```python
from build123d import *

# Parameters (mm, degrees)
SKETCH_1_R       = 2.9
EXTRUDE_1_DEPTH  = 4
CHAMFER_1_SIZE   = 0.6
SKETCH_3_W       = 12
SKETCH_3_H       = 19.86
EXTRUDE_2_DEPTH  = 2
SKETCH_4_W       = 10
SKETCH_4_H       = 12
SKETCH_4_R       = 1.6
EXTRUDE_3_DEPTH  = 3
FILLET_START     = -15
FILLET_2_DEPTH   = 4.14
FILLET_START_2   = -13.86
FILLET_2_2_DEPTH = 3
CHAMFER_4_SIZE   = 1


with BuildPart() as part:
    # 草图1 → 凸台-拉伸1 (new body)
    with BuildSketch(Plane.XY):
        Polygon((7.937253933, 6), (-21, 6), (-21, -13.86), (7.937253933, -13.86), (21, -13.86), (21, 6), align=None)
        Circle(SKETCH_1_R, mode=Mode.SUBTRACT)
    extrude(amount=EXTRUDE_1_DEPTH)

    # 倒角1
    chamfer_1_edges = [part.edges().sort_by_distance(p)[0] for p in [
        (-2.9, 0, 4),
    ]]
    chamfer(chamfer_1_edges, length=CHAMFER_1_SIZE)

    # 草图3 → 凸台-拉伸2 (add)
    with BuildSketch(Plane.ZY.offset(21)):
        with Locations((6, -3.93)):
            Rectangle(SKETCH_3_W, SKETCH_3_H)
    extrude_2 = extrude(amount=EXTRUDE_2_DEPTH)

    # 镜向1: 凸台-拉伸2 across plane
    add(extrude_2.mirror(Plane(origin=(0, 0, 0), x_dir=(0, 0, 1), z_dir=(1, 0, 0))))

    # 草图4 → 凸台-拉伸3 (add)
    # profile 1 of 2: a face of its own
    with BuildSketch(Plane.XZ.offset(13.86)):
        with Locations((-18, 6)):
            Rectangle(SKETCH_4_W, SKETCH_4_H)
        with Locations((-17, 8)):
            Circle(SKETCH_4_R, mode=Mode.SUBTRACT)
    # profile 2 of 2: a face of its own
    with BuildSketch(Plane.XZ.offset(13.86)):
        with Locations((18, 6)):
            Rectangle(SKETCH_4_W, SKETCH_4_H)
        with Locations(Location((17, 8, 0), (0, 0, 180))):
            Circle(SKETCH_4_R, mode=Mode.SUBTRACT)
    extrude(amount=-EXTRUDE_3_DEPTH)

    # 圆角2: read off the stored shape, not the designer's step
    # 圆角2 outline → 圆角2 (cut)
    with BuildSketch(Plane(origin=(0, 0, 0), x_dir=(1, 0, 0), z_dir=(0, 1, 0)).offset(FILLET_START)):
        with BuildLine():
            Line((13, -12), (17, -12))
            ThreePointArc((17, -12), (14.171572875, -10.828427125), (13, -8))
            Line((13, -8), (13, -12))
        make_face()
        with BuildLine():
            Line((-13, -12), (-13, -8))
            ThreePointArc((-13, -8), (-14.171572875, -10.828427125), (-17, -12))
            Line((-17, -12), (-13, -12))
        make_face()
    extrude(amount=FILLET_2_DEPTH, mode=Mode.SUBTRACT)

    # Fillet 2 2 outline → Fillet 2 2 (add)
    with BuildSketch(Plane(origin=(0, 0, 0), x_dir=(1, 0, 0), z_dir=(0, 1, 0)).offset(FILLET_START_2)):
        with BuildLine():
            ThreePointArc((-13, -8), (-11.828427125, -5.171572875), (-9, -4))
            Line((-9, -4), (-13, -4))
            Line((-13, -4), (-13, -8))
        make_face()
        with BuildLine():
            ThreePointArc((9, -4), (11.828427125, -5.171572875), (13, -8))
            Line((13, -8), (13, -4))
            Line((13, -4), (9, -4))
        make_face()
    extrude(amount=FILLET_2_2_DEPTH)

    # 倒角4
    chamfer_4_edges = [part.edges().sort_by_distance(p)[0] for p in [
        (-23, 6, 6),
        (-23, -3.93, 0),
        (-23, -13.86, 6),
        (23, -13.86, 6),
        (23, -3.93, 0),
        (23, 6, 6),
        (0, 6, 0),
        (0, -13.86, 0),
    ]]
    chamfer(chamfer_4_edges, length=CHAMFER_4_SIZE)


solid = part.part
```
Input: part model. Units: mm. Frame: model coordinates. A direction names the side the tool comes from. Give positions to 0.01 mm unless a question says otherwise; leave off trailing zeros. Order: outer loops, then holes, each group sorted by start corner. A loop starts at its lowest first (then second) coordinate and runs counter-clockwise, first axis right, second up. Notation, with made-up numbers: M 88.25,46 L 94.25,46 A7 ccw 94.25,56 Z; hole C 71.5,30.25 d3. An arc over 180 degrees is marked long. Return JSON: item names as keys, results as strings.
1) Line query: L1, parallel to X at y = -9.75, z = 11.25; L2, parallel to Z at x = -17, y = -12; L3, parallel to Y at x = 0, z = 1.05. Output: solid intervals per line, ascending. Write a range as [from, to].
Taken from the geometry:
{"L1": "x = [-23, -21], [21, 23]", "L2": "z = [0, 6.4], [9.6, 12]", "L3": "y = [-13.86, -2.9], [2.9, 6]"}
2) Section query C-C on z = 8.75. Output: boundary loops of the cut face in (x, y).
Taken from the geometry:
{"outline": "M -23,-12.86 L -22,-13.86 L -18.41,-13.86 L -18.41,-10.86 L -21,-10.86 L -21,6 L -22,6 L -23,5 Z; M -15.59,-13.86 L -13.07,-13.86 L -13.07,-10.86 L -15.59,-10.86 Z; M 13.07,-13.86 L 15.59,-13.86 L 15.59,-10.86 L 13.07,-10.86 Z; M 18.41,-13.86 L 22,-13.86 L 23,-12.86 L 23,5 L 22,6 L 21,6 L 21,-10.86 L 18.41,-10.86 Z"}
3) Section query D-D on y = -5.5. Output: boundary loops of the cut face in (x, z), and give its area (3 significant figures).
Taken from the geometry:
{"outline": "M -23,1 L -22,0 L 22,0 L 23,1 L 23,12 L 21,12 L 21,4 L -21,4 L -21,12 L -23,12 Z", "area": "215 mm2"}
4) Mould query, pull axis X, two halves, no side actions, for faces 3 (the face through (21, -2, 8)), 4 (the face through (22.49, -13.37, 6.42)), 5 (the face through (-21.3, -6.3, 12)), 6 (the face through (-2.9, 0.1, 1.7)). Classes: released by +X, released by -X, zero draft, split by the parting line, or undercut.
Taken from the geometry:
{"face 3": "undercut", "face 4": "released by +X", "face 5": "zero draft", "face 6": "undercut"}
5) Access query for faces 1 (the face through (0, -4, 4)), 2 (the face through (21.3, -6.3, 12)). Directions: +Z, -Z, +X, -X, +Y, -Y. A direction counts if a zero-diameter tool reaches every point of the face in a straight line with its end or side. Return the directions, or none.
Taken from the geometry:
{"face 1": "+Z, +Y", "face 2": "+Z, +X, -X, +Y, -Y"}
6) Section query A-A on y = -11.5. Output: boundary loops of the cut face in (x, z).
Taken from the geometry:
{"outline": "M -23,1 L -22,0 L 22,0 L 23,1 L 23,12 L 17,12 A4 ccw 13,8 A4 cw 9,4 L -9,4 A4 cw -13,8 A4 ccw -17,12 L -23,12 Z; hole C -17,8 d3.2; hole C 17,8 d3.2"}
7) Section query B-B on x = 20.5. Output: boundary loops of the cut face in (y, z), and give its area (3 significant figures).
Taken from the geometry:
{"outline": "M -13.86,1 L -12.86,0 L 5,0 L 6,1 L 6,4 L -10.86,4 L -10.86,12 L -13.86,12 Z", "area": "102 mm2"}
8) Contact query for flat-ended pins moving along their axis: pin 1 (6.5 mm diameter, centred on x = -13, z = 10, fed in from +Y); pin 2 (10 mm diameter, centred on x = -10.5, y = -4, fed in from +Z); pin 3 (6.5 mm diameter, centred on x = 0, y = 0, fed in from +Z). Output: stop coordinate, or through.
Taken from the geometry:
{"pin 1": "stops at y = -10.86", "pin 2": "stops at z = 4", "pin 3": "stops at z = 3.75"}
